Model file for the job. Use its own axes, mm. A direction names the side the tool comes from. Give positions to 0.01 mm unless a question says otherwise; leave off trailing zeros. Order: outer loops, then holes, each group sorted by start corner. A loop starts at its lowest first (then second) coordinate and runs counter-clockwise, first axis right, second up. Notation, with made-up numbers: M 41.25,-14 L 51.25,-14 A13 ccw 51.25,9 Z; hole C -37,-5.75 d3. An arc over 180 degrees is marked long. Return JSON: item names as keys, results as strings. Group by question number.
1. Slice it at A-A on x = 5.5. List the corners of the cut face in (y, z).
2. Slice it at B-B on z = -1. List the corners of the cut face in (x, y).
3. Wall check: probe 1 along Y at (x, z) = (0, -0.9); probe 2 along X at (y, z) = (4, -1.15); probe 3 along Y at (x, z) = (4.75, 21.5). Give the ranges that are in metal, low to high. Write a range as [from, to].
4. Pin check, flat tips, straight feed: pin 1 (5 mm diameter, centred on y = 11, z = 12, fed in from -X); pin 2 (5 mm diameter, centred on x = -4.5, z = 9, fed in from -Y); pin 3 (0.9 mm diameter, centred on x = 8, y = 10.5, fed in from +Z); pin 4 (8 mm diameter, centred on x = -3.5, y = 7, fed in from +Z). Stop position of each tip, or through.
5. Slice it at C-C on z = 22. List the corners of the cut face in (x, y).
6. Two-plate mould, pull along X, no slides. Class faces 6 (the face through (8, 11, 16.9)), 7 (the face through (2.37, 2.606, 1.726)), 8 (the face through (7, 12, 20)): released by +X, released by -X, zero draft, split by the parting line, or undercut.
7. 3-axis set-ups, long thin cutter, end or side, ignore diameter. For faces 1 (the face through (2.39, 5.36, 2)), 2 (the face through (0, 6, -3.5)), 3 (the face through (0, 0, 0)), 4 (the face through (5, 8, 14)), 5 (the face through (-2.4, 6, 3.5)): which of +Z, -Z, +X, -X, +Y, -Y reach the whole face in a straight line?
8. Slice it at D-D on y = 11. List the corners of the cut face in (x, z).
from build123d import *

# Parameters (mm, degrees)
ESQUISSE1_W                  = 20
ESQUISSE1_H                  = 7
BOSS_EXTRU_1_DEPTH           = 10
BOSS_EXTRU_2_DEPTH           = 10
ESQUISSE3_W                  = 3
ESQUISSE3_H                  = 9.2
ENL_V_MAT_EXTRU_1_DEPTH      = 30.93743476
ESQUISSE4_R                  = 1.5
ENL_V_MAT_EXTRU_2_DEPTH      = 30.93743476
ENL_V_MAT_EXTRU_4_DEPTH      = 28.147743921
ENL_V_MAT_EXTRU_4_DEPTH_BACK = 28.147743921
ESQUISSE7_R                  = 1.5
ENL_V_MAT_EXTRU_3_DEPTH      = 28.147743921
ENL_V_MAT_EXTRU_3_DEPTH_BACK = 3.5


with BuildPart() as part:
    # Esquisse1 → Boss.-Extru.1 (new body)
    with BuildSketch(Plane(origin=(0, 0, 0), x_dir=(1, 0, 0), z_dir=(0, 1, 0))):
        Rectangle(ESQUISSE1_W, ESQUISSE1_H)
    extrude(amount=BOSS_EXTRU_1_DEPTH)

    # Esquisse2 → Boss.-Extru.2 (add)
    with BuildSketch(Plane(origin=(0, 0, 0), x_dir=(0, 0, -1), z_dir=(1, 0, 0))):
        with BuildLine():
            Line((-3.5, 5), (-3.5, 10))
            Line((-3.5, 10), (0.510302645, 10))
            Line((0.510302645, 10), (-3.489697355, 14))
            Line((-3.489697355, 14), (-21.5, 14))
            ThreePointArc((-21.5, 14), (-24.5, 11), (-21.5, 8))
            Line((-21.5, 8), (-6.5, 8))
            Line((-6.5, 8), (-3.5, 5))
        make_face()
    extrude(amount=BOSS_EXTRU_2_DEPTH)

    # Esquisse3 → Enlèv. mat.-Extru.1 (cut, through all)
    with BuildSketch(Plane(origin=(0, 14, 0), x_dir=(1, 0, 0), z_dir=(0, 1, 0))):
        with Locations((8.5, -21.5)):
            Rectangle(ESQUISSE3_W, ESQUISSE3_H)
    extrude(amount=-ENL_V_MAT_EXTRU_1_DEPTH, mode=Mode.SUBTRACT)

    # Esquisse4 → Enlèv. mat.-Extru.2 (cut, through all)
    with BuildSketch(Plane.ZY):
        with Locations((21.5, 11)):
            Circle(ESQUISSE4_R)
    extrude(amount=-ENL_V_MAT_EXTRU_2_DEPTH, mode=Mode.SUBTRACT)

    # Esquisse7 → Enlèv. mat.-Extru.4 (cut, two sides: drawn at the far end of the back side and taken through both)
    with BuildSketch(Plane.XY.offset(3.5).offset(-ENL_V_MAT_EXTRU_4_DEPTH_BACK)):
        with Locations((0, 4)):
            Circle(ESQUISSE7_R)
    extrude(amount=ENL_V_MAT_EXTRU_4_DEPTH + ENL_V_MAT_EXTRU_4_DEPTH_BACK, mode=Mode.SUBTRACT)

    # Esquisse5 → Enlèv. mat.-Extru.3 (cut, two sides: drawn at the far end of the back side and taken through both)
    with BuildSketch(Plane.XY.offset(3.5).offset(-ENL_V_MAT_EXTRU_3_DEPTH_BACK)):
        Polygon((-1.58771324, 6.75), (-3.175426481, 4), (-1.58771324, 1.25), (1.58771324, 1.25), (3.175426481, 4), (1.58771324, 6.75), align=None)
    extrude(amount=ENL_V_MAT_EXTRU_3_DEPTH + ENL_V_MAT_EXTRU_3_DEPTH_BACK, mode=Mode.SUBTRACT)


solid = part.part
Result:
{
 "1": {"outline": "M 0,-3.5 L 10,-3.5 L 10,-0.51 L 14,3.49 L 14,21.5 A3 ccw 8,21.5 L 8,6.5 L 5,3.5 L 0,3.5 Z; hole C 11,21.5 d3"},
 "2": {"outline": "M -10,0 L 10,0 L 10,10 L -10,10 Z; hole C 0,4 d3"},
 "3": {"probe 1": "y = [0, 2.5], [5.5, 10]", "probe 2": "x = [-10, -1.5], [1.5, 10]", "probe 3": "y = [8, 9.5], [12.5, 14]"},
 "4": {"pin 1": "stops at x = 0", "pin 2": "passes through", "pin 3": "stops at z = 16.9", "pin 4": "stops at z = 23.68"},
 "5": {"outline": "M 0,8.04 L 7,8.04 L 7,9.59 L 0,9.59 Z; M 0,12.41 L 7,12.41 L 7,13.96 L 0,13.96 Z"},
 "6": {"face 6": "zero draft", "face 7": "undercut", "face 8": "released by +X"},
 "7": {"face 1": "+Z", "face 2": "-Z, +X, -X, +Y, -Y", "face 3": "+Z, -Z, +X, -X, -Y", "face 4": "+Z, +X, -X, -Y", "face 5": "+Z, -X, -Y"},
 "8": {"outline": "M 0,0.49 L 10,0.49 L 10,16.9 L 7,16.9 L 7,20 L 0,20 Z; M 0,23 L 7,23 L 7,24.5 L 0,24.5 Z"}
}
